Can you work these out from the model? Positions are in its coordinate system, mm. A direction names the side the tool comes from. Coordinates: 2 decimals unless noted, no trailing zeros. Order: outer loops, then holes, each group sorted by start corner. A loop starts at its lowest first (then second) coordinate and runs counter-clockwise, first axis right, second up. Notation, with made-up numbers: (30.25, 53) -> (71.25, 53) arc R19 cw to (71.25, 59) -> close; hole circle Ø7 at (-37, 23). An arc over 180 degrees is marked (long way). Write item = value, one per line. Start each with the question number.
from build123d import *

# Parameters (mm, degrees)
SKETCH_7_R          = 73.9
EXTRUDE_1_DEPTH     = 5
CUT_EXTRUDE_1_REACH = 229.923
SKETCH_8_R          = 1.6


with BuildPart() as part:
    # Sketch 7 → Extrude 1 (new body)
    with BuildSketch(Plane(origin=(0, 0, 0), x_dir=(1, 0, 0), z_dir=(0, 1, 0))):
        with BuildLine():
            Line((17.737317935, 129.781745931), (-17.737317935, 129.781745931))
            Line((-17.737317935, 129.781745931), (-29.861673588, 150.781745931))
            ThreePointArc((-29.861673588, 150.781745931), (-33.521927626, 154.441999968), (-38.521927626, 155.781745931))
            Line((-38.521927626, 155.781745931), (-117.041564235, 155.781745931))
            ThreePointArc((-117.041564235, 155.781745931), (-122.041564235, 154.441999968), (-125.701818273, 150.781745931))
            Line((-125.701818273, 150.781745931), (-164.961636578, 82.781745931))
            ThreePointArc((-164.961636578, 82.781745931), (-166.30138254, 77.781745931), (-164.961636578, 72.781745931))
            Line((-164.961636578, 72.781745931), (-133.044705684, 17.5))
            ThreePointArc((-133.044705684, 17.5), (-128.355594816, 0), (-133.044705684, -17.5))
            Line((-133.044705684, -17.5), (-164.961636578, -72.781745931))
            ThreePointArc((-164.961636578, -72.781745931), (-166.30138254, -77.781745931), (-164.961636578, -82.781745931))
            Line((-164.961636578, -82.781745931), (-125.701818273, -150.781745931))
            ThreePointArc((-125.701818273, -150.781745931), (-122.041564235, -154.441999968), (-117.041564235, -155.781745931))
            Line((-117.041564235, -155.781745931), (-38.521927626, -155.781745931))
            ThreePointArc((-38.521927626, -155.781745931), (-33.521927626, -154.441999968), (-29.861673588, -150.781745931))
            Line((-29.861673588, -150.781745931), (-17.737317935, -129.781745931))
            Line((-17.737317935, -129.781745931), (17.737317935, -129.781745931))
            Line((17.737317935, -129.781745931), (29.861673588, -150.781745931))
            ThreePointArc((29.861673588, -150.781745931), (33.521927626, -154.441999968), (38.521927626, -155.781745931))
            Line((38.521927626, -155.781745931), (117.041564235, -155.781745931))
            ThreePointArc((117.041564235, -155.781745931), (122.041564235, -154.441999968), (125.701818273, -150.781745931))
            Line((125.701818273, -150.781745931), (164.961636578, -82.781745931))
            ThreePointArc((164.961636578, -82.781745931), (166.30138254, -77.781745931), (164.961636578, -72.781745931))
            Line((164.961636578, -72.781745931), (133.044705684, -17.5))
            ThreePointArc((133.044705684, -17.5), (128.355594816, 0), (133.044705684, 17.5))
            Line((133.044705684, 17.5), (164.961636578, 72.781745931))
            ThreePointArc((164.961636578, 72.781745931), (166.30138254, 77.781745931), (164.961636578, 82.781745931))
            Line((164.961636578, 82.781745931), (125.701818273, 150.781745931))
            ThreePointArc((125.701818273, 150.781745931), (122.041564235, 154.441999968), (117.041564235, 155.781745931))
            Line((117.041564235, 155.781745931), (38.521927626, 155.781745931))
            ThreePointArc((38.521927626, 155.781745931), (33.521927626, 154.441999968), (29.861673588, 150.781745931))
            Line((29.861673588, 150.781745931), (17.737317935, 129.781745931))
        make_face()
        with Locations(Location((77.781745931, 77.781745931, 0), (0, 0, 270))):
            Circle(SKETCH_7_R, mode=Mode.SUBTRACT)
        with Locations(Location((-77.781745931, 77.781745931, 0), (0, 0, 270))):
            Circle(SKETCH_7_R, mode=Mode.SUBTRACT)
        with Locations(Location((-77.781745931, -77.781745931, 0), (0, 0, 270))):
            Circle(SKETCH_7_R, mode=Mode.SUBTRACT)
        with Locations(Location((77.781745931, -77.781745931, 0), (0, 0, 270))):
            Circle(SKETCH_7_R, mode=Mode.SUBTRACT)
        with BuildLine():
            Line((10.231764435, 125.781745931), (-10.231764435, 125.781745931))
            ThreePointArc((-10.231764435, 125.781745931), (-12.829840647, 124.281745931), (-12.829840647, 121.281745931))
            Line((-12.829840647, 121.281745931), (-8.660254038, 114.059810077))
            ThreePointArc((-8.660254038, 114.059810077), (0, 109.059810077), (8.660254038, 114.059810077))
            Line((8.660254038, 114.059810077), (12.829840647, 121.281745931))
            ThreePointArc((12.829840647, 121.281745931), (12.829840647, 124.281745931), (10.231764435, 125.781745931))
        make_face(mode=Mode.SUBTRACT)
        with BuildLine():
            Line((12.829840647, -121.281745931), (8.660254038, -114.059810077))
            ThreePointArc((8.660254038, -114.059810077), (0, -109.059810077), (-8.660254038, -114.059810077))
            Line((-8.660254038, -114.059810077), (-12.829840647, -121.281745931))
            ThreePointArc((-12.829840647, -121.281745931), (-12.829840647, -124.281745931), (-10.231764435, -125.781745931))
            Line((-10.231764435, -125.781745931), (10.231764435, -125.781745931))
            ThreePointArc((10.231764435, -125.781745931), (12.829840647, -124.281745931), (12.829840647, -121.281745931))
        make_face(mode=Mode.SUBTRACT)
    extrude(amount=EXTRUDE_1_DEPTH)

    # Sketch 8 → Cut-Extrude 1 (cut, up to next)
    with BuildSketch(Plane(origin=(0, 5, 0), x_dir=(1, 0, 0), z_dir=(0, 1, 0)), mode=Mode.PRIVATE) as cut_extrude_1_sk1:
        with Locations(Location((80, 0, 0), (0, 0, 270))):
            Circle(SKETCH_8_R)
    cut_extrude_1_tool1 = extrude(cut_extrude_1_sk1.sketch, amount=-CUT_EXTRUDE_1_REACH, mode=Mode.PRIVATE) & part.part
    # Sketch 8 → Cut-Extrude 1 (cut, up to next)
    with BuildSketch(Plane(origin=(0, 5, 0), x_dir=(1, 0, 0), z_dir=(0, 1, 0)), mode=Mode.PRIVATE) as cut_extrude_1_sk2:
        with Locations(Location((0, -80, 0), (0, 0, 270))):
            Circle(SKETCH_8_R)
    cut_extrude_1_tool2 = extrude(cut_extrude_1_sk2.sketch, amount=-CUT_EXTRUDE_1_REACH, mode=Mode.PRIVATE) & part.part
    # Sketch 8 → Cut-Extrude 1 (cut, up to next)
    with BuildSketch(Plane(origin=(0, 5, 0), x_dir=(1, 0, 0), z_dir=(0, 1, 0)), mode=Mode.PRIVATE) as cut_extrude_1_sk3:
        with Locations(Location((-80, 0, 0), (0, 0, 270))):
            Circle(SKETCH_8_R)
    cut_extrude_1_tool3 = extrude(cut_extrude_1_sk3.sketch, amount=-CUT_EXTRUDE_1_REACH, mode=Mode.PRIVATE) & part.part
    # Sketch 8 → Cut-Extrude 1 (cut, up to next)
    with BuildSketch(Plane(origin=(0, 5, 0), x_dir=(1, 0, 0), z_dir=(0, 1, 0)), mode=Mode.PRIVATE) as cut_extrude_1_sk4:
        with Locations(Location((0, 80, 0), (0, 0, 270))):
            Circle(SKETCH_8_R)
    cut_extrude_1_tool4 = extrude(cut_extrude_1_sk4.sketch, amount=-CUT_EXTRUDE_1_REACH, mode=Mode.PRIVATE) & part.part
    # Sketch 8 → Cut-Extrude 1 (cut, up to next)
    with BuildSketch(Plane(origin=(0, 5, 0), x_dir=(1, 0, 0), z_dir=(0, 1, 0)), mode=Mode.PRIVATE) as cut_extrude_1_sk5:
        with BuildLine():
            ThreePointArc((0, 59.073458997), (21.213203436, 21.213203436), (59.073458997, 0))
            ThreePointArc((59.073458997, 0), (21.213203436, -21.213203436), (0, -59.073458997))
            ThreePointArc((0, -59.073458997), (-21.213203436, -21.213203436), (-59.073458997, 0))
            ThreePointArc((-59.073458997, 0), (-21.213203436, 21.213203436), (0, 59.073458997))
        make_face()
    cut_extrude_1_tool5 = extrude(cut_extrude_1_sk5.sketch, amount=-CUT_EXTRUDE_1_REACH, mode=Mode.PRIVATE) & part.part
    add(cut_extrude_1_tool1.solids().sort_by_distance((80, 5, 0))[0], mode=Mode.SUBTRACT)
    add(cut_extrude_1_tool2.solids().sort_by_distance((0, 5, 80))[0], mode=Mode.SUBTRACT)
    add(cut_extrude_1_tool3.solids().sort_by_distance((-80, 5, 0))[0], mode=Mode.SUBTRACT)
    add(cut_extrude_1_tool4.solids().sort_by_distance((0, 5, -80))[0], mode=Mode.SUBTRACT)
    add(cut_extrude_1_tool5.solids().sort_by_distance((0, 5, 0))[0], mode=Mode.SUBTRACT)


solid = part.part
(1) For faces 1 (the face through (23.884, 2.465, -140.429)), 2 (the face through (-23.884, 2.465, 140.429)), 3 (the face through (-148.78, 2.465, 44.754)), 4 (the face through (-143.344, 2.465, -43.681)), 5 (the face through (149.23, 2.46, 45.53)), which set-ups out of +Z, -Z, +X, -X, +Y, -Y let a thin tool reach every point of the face, with its end or its side?
(2) Thinking about a two-plate mould opening in Z: for faces 6 (the face through (-20.78, 2.54, 21.65)), 7 (the face through (23.71, 2.46, 140.13)), 8 (the face through (145.607, 2.465, -116.306)), which applies, +Z half, -Z half, draft (parallel to the pull), parting line (faces both ways), or undercut?
(3) If I drill on L1, parallel to Z at x = -80, y = 1.15; L2, parallel to Z at x = 75, y = 3.35; L3, parallel to X at y = 3, z = -86, over which ranges is the centre line in solid material (lowest first)? Write a range as from..to.
(4) Imagine slicing it at B-B (x = -70). Write out the boundary of the cut face in (y, z), plus the area to 3 significant figures.
(5) Imagine slicing it at D-D (x = 140.5). Write out the boundary of the cut face in (y, z).
(6) Imagine slicing it at C-C (y = 3.7). Count the separate pieces of the cut face and the enclosed holes in it, plus the area to 3 significant figures.
(7) For P1, Ø2.5, axis at x = -3, y = 1.5, coming from the -Z side; P2, Ø2, axis at y = 1.5, z = 1.5, coming from the +X side (3 decimals); P3, Ø1.5, axis at y = 4.5, z = 60.5, coming from the -X side; P4, Ø3, axis at x = 0, z = -80, coming from the +Y side, each with a flat end and sliding along its axis, tell me the tip position at first contact or that it passes through.
(8) Imagine slicing it at A-A (x = 46). Write out the boundary of the cut face in (y, z), plus the area to 3 significant figures.
Result set:
q1.face_1 = -Z, +Y, -Y
q1.face_2 = +Z, +Y, -Y
q1.face_3 = -X, +Y, -Y
q1.face_4 = +Y, -Y
q1.face_5 = +X, +Y, -Y
q2.face_6 = undercut
q2.face_7 = +Z half
q2.face_8 = -Z half
q3.L1 = -155.78..-151.65, -3.92..-1.6, 1.6..3.92, 151.65..155.78
q3.L2 = -155.78..-151.63, -3.93..3.93, 151.63..155.78
q3.L3 = -163.1..-151.22, -4.34..4.34, 151.22..163.1
q4.outline = (0, -155.78) -> (5, -155.78) -> (5, -151.27) -> (0, -151.27) -> close; (0, -4.29) -> (5, -4.29) -> (5, 4.29) -> (0, 4.29) -> close; (0, 151.27) -> (5, 151.27) -> (5, 155.78) -> (0, 155.78) -> close
q4.area = 88.0 mm2
q5.outline = (0, -125.15) -> (5, -125.15) -> (5, -116.87) -> (0, -116.87) -> close; (0, -38.7) -> (5, -38.7) -> (5, -30.41) -> (0, -30.41) -> close; (0, 30.41) -> (5, 30.41) -> (5, 38.7) -> (0, 38.7) -> close; (0, 116.87) -> (5, 116.87) -> (5, 125.15) -> (0, 125.15) -> close
q6.separate_pieces = 1
q6.enclosed_holes = 11
q6.area = 14,400 mm2
q7.P1 = -129.78
q7.P2 = 128.445
q7.P3 = -158.3
q7.P4 = through
q8.outline = (0, -155.78) -> (5, -155.78) -> (5, -144.5) -> (0, -144.5) -> close; (0, -11.06) -> (5, -11.06) -> (5, -4.37) -> (0, -4.37) -> close; (0, 4.37) -> (5, 4.37) -> (5, 11.06) -> (0, 11.06) -> close; (0, 144.5) -> (5, 144.5) -> (5, 155.78) -> (0, 155.78) -> close
q8.area = 180 mm2
